Here's how the part is built. I have some questions about the finished solid (model axes, mm). A direction names the side the tool comes from. Coordinates: 2 decimals unless noted, no trailing zeros. Write each loop counter-clockwise with the first axis right and the second up, starting at its lowest first coordinate (ties: lowest second). Pieces come first, ordered by that corner, then holes. Notation, with made-up numbers: (20.5, -9.75) - (61.5, -9.75) arc R21 cw to (61.5, 3.25) - close; hole circle Ø2 at (36, 12.25). An arc over 180 degrees is marked (long way). Answer in a Markdown table with one row per item. Add a question column.
Item 1: Imagine slicing it at D-D (x = -48). Please give me the cut outline in (y, z).
Item 2: Imagine slicing it at B-B (x = -5.5). Please give me the cut outline in (y, z), plus the area to 3 significant figures.
Item 3: Imagine slicing it at A-A (z = 2). Please give me the cut outline in (x, y), plus the area to 3 significant figures.
Item 4: If I drill on probe 1 along Y at (x, z) = (-14, 6.5); probe 2 along X at (y, z) = (0.5, 1); probe 3 along Y at (x, z) = (-22, 3.75), over which ranges is the centre line in solid material (lowest first)? Write a range as from..to.
Item 5: Imagine slicing it at C-C (z = 6). Please give me the cut outline in (x, y), plus the area to 3 significant figures.
Item 6: We'd pull the mould along Y, two halves only. Please class faces 5 (the face through (-35, 2, 7)), 6 (the face through (-63.326, 14.599, 3.549)), 7 (the face through (-35, 9, 5)): +Y half, -Y half, draft (parallel to the pull), parting line (faces both ways), or undercut.
Item 7: Which directions (+Z, -Z, +X, -X, +Y, -Y) give clear straight access to the entire face, cutting with the end or side of a thin tool? Please do faces 1 (the face through (-4.83, 10, 3)), 2 (the face through (-66.2, 2.4, 3)), 3 (the face through (-64.83, 10, 3)), 4 (the face through (-35, 1.024, 3)).
Item 8: I'm going to push flat-ended pins straight in: pin 1 (1.5 mm diameter, centred on y = 8, z = 1, fed in from +X); pin 2 (0.7 mm diameter, centred on y = 10, z = 5, fed in from +X); pin 3 (2 mm diameter, centred on x = -64.83, y = 1.02, fed in from +Z); pin 4 (1.5 mm diameter, centred on y = -0.5, z = 5, fed in from -X). Where does each tip first touch, or does it pass through?
Autodesk Fusion 360 part; units mm, degrees
sketch "Sketch1" plane through (0, 0, 0) normal (0, 0, 1) x (1, 0, 0) in component "node_nametag"
  circle A0 centre (-64.8296, 1.0244) radius 1.75
  circle A1 centre (-4.8296, 1.0244) radius 1.75
  circle A2 centre (-64.8296, 1.0244) radius 5
  circle A3 centre (-4.8296, 1.0244) radius 5
  line L0 (-64.8296, 16.0244) -> (-4.8296, 16.0244)
  line L1 (-4.8296, 16.0244) -> (-4.8296, 1.0244)
  line L2 (-4.8296, 1.0244) -> (-64.8296, 1.0244)
  line L3 (-64.8296, 1.0244) -> (-64.8296, 16.0244)
  dimension "d1" = 3.5
  dimension "d2" = 3.5
  dimension "d3" = 60
  dimension "d4" = 10
  dimension "d5" = 10
  dimension "d6" = 15
extrude "Extrude1" add sketch "Sketch1" along normal blind 5 contours A0 A2 L2 L3 | A0 A2 L2 L3 | A2 A3 L0 L1 L2 L3 | A1 A3 L1 L2 | A1 A3 L1 L2 in component "node_nametag"
sketch "Sketch2" plane through (0, 0, 5) normal (0, 0, 1) x (-1, 0, 0) in component "node_nametag"
  circle A0 centre (4.8296, -1.0244) radius 1.75
  circle A1 centre (64.8296, -1.0244) radius 1.75
  line L0 (64.8296, -16.0244) -> (64.8296, -6.0244)
  arc A2 (64.8296, -6.0244) -> (59.8296, -1.0244) centre (64.8296, -1.0244) ccw
  line L1 (59.8296, -1.0244) -> (9.8296, -1.0244)
  arc A3 (9.8296, -1.0244) -> (4.8296, -6.0244) centre (4.8296, -1.0244) ccw
  line L2 (4.8296, -6.0244) -> (4.8296, -16.0244)
  line L3 (4.8296, -16.0244) -> (64.8296, -16.0244)
  line L4 (62.3296, -14.5244) -> (7.3296, -14.5244)
  line L5 (7.3296, -14.5244) -> (7.3296, -2.5244)
  line L6 (7.3296, -2.5244) -> (62.3296, -2.5244)
  line L7 (62.3296, -2.5244) -> (62.3296, -14.5244)
  line L8 (34.8296, -16.0244) -> (34.8296, -1.0244) construction
  line L9 (64.8296, -11.0244) -> (4.8296, -11.0244) construction
  dimension "d9" = 12
  dimension "d10" = 55
  dimension "d11" = 27.5
  dimension "d12" = 1.5
extrude "Extrude2" add sketch "Sketch2" along normal blind 2 in component "node_nametag"
fillet "Fillet1" radius 5 6 edges at (-4.8296, 16.0244, 3.5) (-64.8296, 16.0244, 3.5) (-59.8296, 1.0244, 3.5) (-9.8296, 1.0244, 3.5) (-64.8296, 6.0244, 3.5) (-4.8296, 6.0244, 3.5) in component "node_nametag"
fillet "Fillet1" radius 2 4 edges at (-62.3296, 14.5244, 6) (-62.3296, 2.5244, 6) (-7.3296, 2.5244, 6) (-7.3296, 14.5244, 6) in component "node_nametag"
sketch "Sketch3" plane through (0, 0, 7) normal (0, 0, 1) x (-1, 0, 0) in component "node_nametag"
  line L0 (9.3296, -2.5244) -> (60.3296, -2.5244)
  arc A0 (62.3296, -4.5244) -> (60.3296, -2.5244) centre (60.3296, -4.5244) ccw
  line L1 (62.3296, -4.5244) -> (62.3296, -12.5244)
  arc A1 (60.3296, -14.5244) -> (62.3296, -12.5244) centre (60.3296, -12.5244) ccw
  line L2 (60.3296, -14.5244) -> (9.3296, -14.5244)
  arc A2 (7.3296, -12.5244) -> (9.3296, -14.5244) centre (9.3296, -12.5244) ccw
  line L3 (7.3296, -12.5244) -> (7.3296, -4.5244)
  arc A3 (9.3296, -2.5244) -> (7.3296, -4.5244) centre (9.3296, -4.5244) ccw
  circle A4 centre (4.8296, -1.0244) radius 1.75
  circle A5 centre (64.8296, -1.0244) radius 1.75
  arc A6 (59.8296, -16.0244) -> (64.8296, -11.0244) centre (59.8296, -11.0244) ccw
  line L4 (64.8296, -11.0244) -> (64.8296, -9.6847)
  arc A7 (67.3296, -5.3546) -> (64.8296, -9.6847) centre (69.8296, -9.6847) ccw
  arc A8 (67.3296, -5.3546) -> (60.4995, 1.4756) centre (64.8296, -1.0244) ccw
  arc A9 (56.1694, -1.0244) -> (60.4995, 1.4756) centre (56.1694, 3.9756) ccw
  line L5 (56.1694, -1.0244) -> (13.4899, -1.0244)
  arc A10 (9.1597, 1.4756) -> (13.4899, -1.0244) centre (13.4899, 3.9756) ccw
  arc A11 (9.1597, 1.4756) -> (2.3296, -5.3546) centre (4.8296, -1.0244) ccw
  arc A12 (4.8296, -9.6847) -> (2.3296, -5.3546) centre (-0.1704, -9.6847) ccw
  line L6 (4.8296, -9.6847) -> (4.8296, -11.0244)
  arc A13 (4.8296, -11.0244) -> (9.8296, -16.0244) centre (9.8296, -11.0244) ccw
  line L7 (9.8296, -16.0244) -> (59.8296, -16.0244)
  circle A14 centre (4.8296, -1.0244) radius 3.25
  circle A15 centre (64.8296, -1.0244) radius 3.25
  dimension "d19" = 6.5
  dimension "d20" = 6.5
extrude "Extrude3" cut sketch "Sketch3" against normal blind 4 contours A14 | A15 in component "node_nametag"
component "node_nametag" placed x (1, 0, 0) y (0, 1, 0) z (0, 0, 1) at (0, 0, 0)
equation "d3 = ( 15 * 4 ) * 1 mm"
equation "d11 = d10 / 2"
Here are the results:
| question | item | result |
|---|---|---|
| 1 | outline | (1.02, 0) - (16.02, 0) - (16.02, 7) - (14.52, 7) - (14.52, 5) - (2.52, 5) - (2.52, 7) - (1.02, 7) - close |
| 2 | outline | (-3.93, 0) - (-0.59, 0) - (-0.59, 3) - (-2.16, 3) - (-2.16, 7) - (-3.93, 7) - close; (2.64, 0) - (13.53, 0) - (13.53, 7) - (4.2, 7) - (4.2, 3) - (2.64, 3) - close |
| 2 | area | 87.1 mm2 |
| 3 | outline | (-67.33, 5.35) arc R5 ccw (long way) to (-60.5, -1.48) arc R5 cw to (-56.17, 1.02) - (-13.49, 1.02) arc R5 cw to (-9.16, -1.48) arc R5 ccw (long way) to (-2.33, 5.35) arc R5 cw to (-4.83, 9.68) - (-4.83, 11.02) arc R5 ccw to (-9.83, 16.02) - (-59.83, 16.02) arc R5 ccw to (-64.83, 11.02) - (-64.83, 9.68) arc R5 cw to start; hole circle Ø3.5 at (-64.83, 1.02); hole circle Ø3.5 at (-4.83, 1.02) |
| 3 | area | 996 mm2 |
| 4 | probe 1 | y = 1.02..2.52, 14.52..16.02 |
| 4 | probe 2 | x = -69.8..-66.5, -63.16..-58.4, -11.26..-6.5, -3.16..0.14 |
| 4 | probe 3 | y = 1.02..16.02 |
| 5 | outline | (-67.33, 5.35) arc R5 ccw (long way) to (-60.5, -1.48) arc R5 cw to (-56.17, 1.02) - (-13.49, 1.02) arc R5 cw to (-9.16, -1.48) arc R5 ccw (long way) to (-2.33, 5.35) arc R5 cw to (-4.83, 9.68) - (-4.83, 11.02) arc R5 ccw to (-9.83, 16.02) - (-59.83, 16.02) arc R5 ccw to (-64.83, 11.02) - (-64.83, 9.68) arc R5 cw to start; hole circle Ø6.5 at (-64.83, 1.02); hole (-62.33, 4.52) arc R2 ccw to (-60.33, 2.52) - (-9.33, 2.52) arc R2 ccw to (-7.33, 4.52) - (-7.33, 12.52) arc R2 ccw to (-9.33, 14.52) - (-60.33, 14.52) arc R2 ccw to (-62.33, 12.52) - close; hole circle Ø6.5 at (-4.83, 1.02) |
| 5 | area | 292 mm2 |
| 6 | face 5 | draft |
| 6 | face 6 | +Y half |
| 6 | face 7 | undercut |
| 7 | face 1 | +Z, -Z, +X, +Y |
| 7 | face 2 | +Z |
| 7 | face 3 | +Z, -Z, -X, +Y |
| 7 | face 4 | +Z, -Z, -Y |
| 8 | pin 1 | stops at x = -4.2 |
| 8 | pin 2 | stops at x = -4.83 |
| 8 | pin 3 | passes through |
| 8 | pin 4 | stops at x = -69.77 |
